```python
from build123d import *

# Parameters (mm, degrees)
SKETCH1_W           = 30.48
SKETCH1_H           = 25.908
BOSS_EXTRUDE1_DEPTH = 5.334
SKETCH2_W           = 20.828
SKETCH2_H           = 20.828
CUT_EXTRUDE1_DEPTH  = 4.572
SKETCH3_W           = 30.48
SKETCH3_H           = 25.908
SKETCH3_W_2         = 17.78
SKETCH3_H_2         = 17.78
BOSS_EXTRUDE2_DEPTH = 0.762
SKETCH4_W           = 2.54
SKETCH4_H           = 12.7
CUT_EXTRUDE5_DEPTH  = 21.909924247


with BuildPart() as part:
    # Sketch1 → Boss-Extrude1 (new body)
    with BuildSketch(Plane.XY):
        Rectangle(SKETCH1_W, SKETCH1_H)
    extrude(amount=BOSS_EXTRUDE1_DEPTH)

    # Sketch2 → Cut-Extrude1 (cut)
    with BuildSketch(Plane.XY.offset(5.334)):
        Rectangle(SKETCH2_W, SKETCH2_H)
    extrude(amount=-CUT_EXTRUDE1_DEPTH, mode=Mode.SUBTRACT)

    # Sketch3 → Boss-Extrude2 (add)
    with BuildSketch(Plane.XY.offset(5.334)):
        Rectangle(SKETCH3_W, SKETCH3_H)
        Rectangle(SKETCH3_W_2, SKETCH3_H_2, mode=Mode.SUBTRACT)
    extrude(amount=BOSS_EXTRUDE2_DEPTH)

    # Sketch4 → Cut-Extrude5 (cut, through all)
    with BuildSketch(Plane.XY.offset(6.096)):
        with Locations((-12.827, 0)):
            Rectangle(SKETCH4_W, SKETCH4_H)
        with Locations((12.827, 0)):
            Rectangle(SKETCH4_W, SKETCH4_H)
    extrude(amount=-CUT_EXTRUDE5_DEPTH, mode=Mode.SUBTRACT)


solid = part.part
```
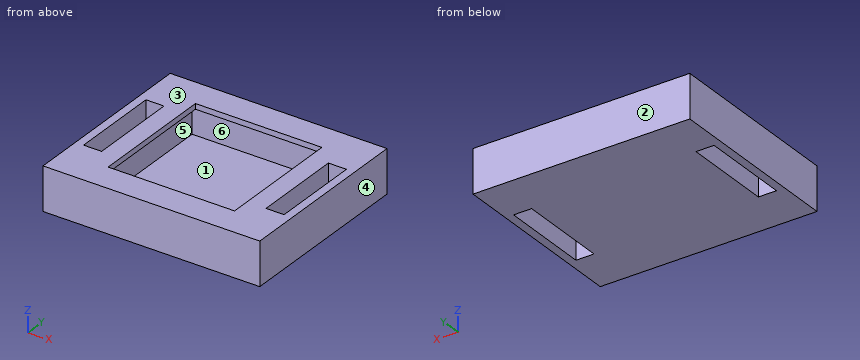
Geometry check sheet. Reference: the model listing, model coordinates, mm. Face numbers are marked on the shaded views. A direction names the side the tool comes from. Coordinates: 2 decimals unless noted, no trailing zeros. Write each loop counter-clockwise with the first axis right and the second up, starting at its lowest first coordinate (ties: lowest second). Pieces come first, ordered by that corner, then holes. Notation, with made-up numbers: M -2.75,33.5 L 27.25,33.5 A26 ccw 27.25,52.5 Z; hole C 46.5,22.5 d11. An arc over 180 degrees is marked long. Use one line per item in the form item = value. Start each with the question number.
1) Section check C-C on z = 3.5. Enter the section's corners in (x, y), and give its area (3 significant figures).
2) Section check B-B on y = 0. Enter the section's corners in (x, z).
3) Thickness scan on probe 1 along X at (y, z) = (1.75, 3.5); probe 2 along X at (y, z) = (-2.75, 5.75); probe 3 along Y at (x, z) = (13, 1.75). Record the ranges inside material, lowest first. Write a range as from..to.
4) Release check for a two-part mould opening along Z. For the marked faces 3, 4, 5 and 6 record: pulls with the +Z half, pulls with the -Z half, needs draft (parallel to the pull), parting line crosses it, or undercut.
5) Section check A-A on x = -12. Enter the section's corners in (y, z), and give its area (3 significant figures).
6) Set-up check for the marked faces 1 and 2: record each of +Z, -Z, +X, -X, +Y, -Y from which the full face is reachable in a straight line by a thin tool's end or side.
7) Section check D-D on y = 8.5. Enter the section's corners in (x, z).
Responses:
q1.outline = M -15.24,-12.95 L 15.24,-12.95 L 15.24,12.95 L -15.24,12.95 Z; hole M -14.1,-6.35 L -11.56,-6.35 L -11.56,6.35 L -14.1,6.35 Z; hole M -10.41,-10.41 L 10.41,-10.41 L 10.41,10.41 L -10.41,10.41 Z; hole M 11.56,-6.35 L 14.1,-6.35 L 14.1,6.35 L 11.56,6.35 Z
q1.area = 291 mm2
q2.outline = M -15.24,0 L -14.1,0 L -14.1,6.1 L -15.24,6.1 Z; M -11.56,0 L 11.56,0 L 11.56,6.1 L 8.89,6.1 L 8.89,5.33 L 10.41,5.33 L 10.41,0.76 L -10.41,0.76 L -10.41,5.33 L -8.89,5.33 L -8.89,6.1 L -11.56,6.1 Z; M 14.1,0 L 15.24,0 L 15.24,6.1 L 14.1,6.1 Z
q3.probe_1 = -15.24..-14.1, -11.56..-10.41, 10.41..11.56, 14.1..15.24
q3.probe_2 = -15.24..-14.1, -11.56..-8.89, 8.89..11.56, 14.1..15.24
q3.probe_3 = -12.95..-6.35, 6.35..12.95
q4.face_3 = pulls with the +Z half
q4.face_4 = needs draft
q4.face_5 = undercut
q4.face_6 = undercut
q5.outline = M -12.95,0 L -6.35,0 L -6.35,6.1 L -12.95,6.1 Z; M 6.35,0 L 12.95,0 L 12.95,6.1 L 6.35,6.1 Z
q5.area = 80.5 mm2
q6.face_1 = none
q6.face_2 = +Z, -Z, +X, -X, +Y
q7.outline = M -15.24,0 L 15.24,0 L 15.24,6.1 L 8.89,6.1 L 8.89,5.33 L 10.41,5.33 L 10.41,0.76 L -10.41,0.76 L -10.41,5.33 L -8.89,5.33 L -8.89,6.1 L -15.24,6.1 Z
